Build history of the part. All positions in model axes, mm. A direction names the side the tool comes from. Coordinates: 2 decimals unless noted, no trailing zeros. Loops run counter-clockwise (first coordinate to the right, second up) from the corner with the lowest first, then second, coordinate; pieces in that order, holes last. Notation, with made-up numbers: (61.25, 16.25) - (119.25, 16.25) arc R30 cw to (119.25, 47.25) - close; hole circle Ø3 at (40.5, -5). An arc over 180 degrees is marked (long way). One line per item, written item: value.
```python
from build123d import *

# Parameters (mm, degrees)
SKETCH1_R           = 1.875
BOSS_EXTRUDE1_DEPTH = 5
BOSS_EXTRUDE2_DEPTH = 12
BOSS_EXTRUDE3_DEPTH = 5
CHAMFER1_SIZE       = 2


with BuildPart() as part:
    # Sketch1 → Boss-Extrude1 (new body)
    with BuildSketch(Plane(origin=(0, 0, 0), x_dir=(1, 0, 0), z_dir=(0, 1, 0))):
        Polygon((-12.5, 50), (12.5, 50), (22.5, 40), (22.5, -50), (-22.5, -50), (-22.5, 40), align=None)
        with Locations(Location((0, 25, 0), (0, 0, 270))):
            Circle(SKETCH1_R, mode=Mode.SUBTRACT)
        with Locations(Location((0, -25, 0), (0, 0, 270))):
            Circle(SKETCH1_R, mode=Mode.SUBTRACT)
    extrude(amount=BOSS_EXTRUDE1_DEPTH)

    # Sketch3 → Boss-Extrude2 (add)
    with BuildSketch(Plane.XZ):
        Polygon((-22.5, 50), (-18.75, 50), (-18.75, -40), (-12.5, -46.25), (12.5, -46.25), (18.75, -40), (18.75, 50), (22.5, 50), (22.5, -40), (12.5, -50), (-12.5, -50), (-22.5, -40), align=None)
    extrude(amount=BOSS_EXTRUDE2_DEPTH)

    # Sketch4 → Cut-Revolve1 (revolve, cut)
    with BuildSketch(Plane(origin=(0, 0, 0), x_dir=(0, 0, -1), z_dir=(1, 0, 0))):
        Polygon((-26.875, 5), (-26.875, 4.3), (-29.5, 0), (-25.875, 0), (-25.875, 5), align=None)
    cut_revolve1 = revolve(axis=Axis((0, 5, 25), (0, -1, 0)), mode=Mode.SUBTRACT)

    # Mirror1: Cut-Revolve1 across plane
    add(cut_revolve1.mirror(Plane.XY), mode=Mode.SUBTRACT)

    # Sketch5 → Boss-Extrude3 (add)
    with BuildSketch(Plane.XZ.offset(12)):
        Polygon((-22.5, -40), (-12.5, -50), (12.5, -50), (22.5, -40), (22.5, 50), (6, 50), (6, -41.25), (-6, -41.25), (-6, 50), (-22.5, 50), align=None)
    extrude(amount=BOSS_EXTRUDE3_DEPTH)

    # Chamfer1
    chamfer1_edges = [part.edges().sort_by_distance(p)[0] for p in [
        (18.75, -12, 5),
        (15.625, -12, -43.125),
        (0, -12, -46.25),
        (-15.625, -12, -43.125),
        (-18.75, -12, 5),
    ]]
    chamfer(chamfer1_edges, length=CHAMFER1_SIZE)


solid = part.part
```
Item 1: Cut at C-C, the plane y = 3. Write the cut outline in (x, z), then the cut area to 3 significant figures.
Check result:
outline: (-22.5, -40) - (-12.5, -50) - (12.5, -50) - (22.5, -40) - (22.5, 50) - (-22.5, 50) - close; hole circle Ø5.34 at (0, -25); hole circle Ø5.34 at (0, 25)
area: 4,360 mm^2
Item 2: Pull direction Y, two halves, no side cores. Call faces 4 (the face through (-0.1, 3.6, 22.7)), 5 (the face through (17.76, -10.99, 4.37)), 6 (the face through (22.5, -6, 4)): released by +Y, released by -Y, zero draft, split by the parting line, or undercut.
Check result:
face 4: released by -Y
face 5: undercut
face 6: zero draft
Item 3: Drop flat-ended pins along their axis: P1, Ø3, axis at x = 9.5, y = -9.5, coming from the +Z side; P2, Ø4, axis at x = 1, y = -14, coming from the +Z side; P3, Ø4.5, axis at x = 0, z = 25, coming from the -Y side; P4, Ø2, axis at x = 0, z = -25, coming from the +Y side. Give the stop position or say it passes through.
Check result:
P1: stops at z = -45.25
P2: stops at z = -41.25
P3: stops at y = 3.69
P4: passes through
Item 4: Cut at B-B, the plane z = -25. Write the cut outline in (x, y) (3 decimals).
Check result:
outline: (-22.5, -17) - (-6, -17) - (-6, -12) - (-16.75, -12) - (-18.75, -10) - (-18.75, 0) - (-4.5, 0) - (-1.875, 4.3) - (-1.875, 5) - (-22.5, 5) - close; (1.875, 4.3) - (4.5, 0) - (18.75, 0) - (18.75, -10) - (16.75, -12) - (6, -12) - (6, -17) - (22.5, -17) - (22.5, 5) - (1.875, 5) - close
Item 5: Cut at D-D, the plane z = 40. Write the cut outline in (x, y).
Check result:
outline: (-22.5, -17) - (-6, -17) - (-6, -12) - (-16.75, -12) - (-18.75, -10) - (-18.75, 0) - (18.75, 0) - (18.75, -10) - (16.75, -12) - (6, -12) - (6, -17) - (22.5, -17) - (22.5, 5) - (-22.5, 5) - close
Item 6: Probe probe 1 along Z at (x, y) = (0, 4.6) (3 decimals); probe 2 along X at (y, z) = (4.8, 25) (3 decimals); probe 3 along Y at (x, z) = (14.5, 7). List the from-to ranges inside material, lowest first. Write a range as from..to.
Check result:
probe 1: z = -50..-26.875, -23.125..23.125, 26.875..50
probe 2: x = -22.5..-1.875, 1.875..22.5
probe 3: y = -17..-12, 0..5
Item 7: Cut at A-A, the plane x = 0. Write the cut outline in (y, z) (3 decimals), then the cut area to 3 significant figures.
Check result:
outline: (-17, -50) - (5, -50) - (5, -26.875) - (4.3, -26.875) - (0, -29.5) - (0, -46.25) - (-10, -46.25) - (-12, -44.25) - (-12, -41.25) - (-17, -41.25) - close; (0, -20.5) - (4.3, -23.125) - (5, -23.125) - (5, 23.125) - (4.3, 23.125) - (0, 20.5) - close; (0, 29.5) - (4.3, 26.875) - (5, 26.875) - (5, 50) - (0, 50) - close
area: 531 mm^2
Item 8: Tool access for faces 1 (the face through (0.56, 4.65, 26.79)), 2 (the face through (-15.67, -4.93, -43.08)), 3 (the face through (-6, -14, 4)): list every direction of +Z, -Z, +X, -X, +Y, -Y with a clear straight run to the whole face (end or side of a thin tool).
Check result:
face 1: +Y, -Y
face 2: +Z
face 3: +Z, -Y
